Autodesk Inventor part; units mm, degrees
ref_plane "YZ Plane" through (0, 0, 0) normal (1, 0, 0) x (0, 1, 0)
ref_plane "XZ Plane" through (0, 0, 0) normal (0, 1, 0) x (-1, 0, 0)
ref_plane "XY Plane" through (0, 0, 0) normal (0, 0, 1) x (1, 0, 0)
sketch "スケッチ1" plane through (0, 0, 0) normal (0, 1, 0) x (-1, 0, 0)
  arc A0 (72.9254, -25.3463) -> (139.4294, -19.0858) centre (64.9013, 416.2515) ccw
  arc A1 (54.1052, -25.1311) -> (72.9254, -25.3463) centre (67.1484, 292.5868) ccw
  arc A2 (19.6951, -19.0145) -> (54.1052, -25.1311) centre (59.4352, 104.7024) ccw
  arc A3 (-0.0609, -9.311) -> (19.6951, -19.0145) centre (42.8692, 53.13) ccw
  arc A4 (-5.5029, -4.0266) -> (-0.0609, -9.311) centre (12.76, 9.3368) ccw
  arc A5 (-2.9938, 3.6874) -> (-5.5029, -4.0266) centre (-1.4678, -1.074) ccw
  arc A6 (5.1717, 4.7562) -> (-2.9938, 3.6874) centre (4.0256, -18.2153) ccw
  arc A7 (36.109, -0.9508) -> (5.1717, 4.7562) centre (-0.7578, -114.096) ccw
  arc A8 (36.109, -0.9508) -> (38.0145, -1.5673) centre (185.125, 456.3841) ccw
  arc A9 (38.0145, -1.5673) -> (139.3334, -17.8944) centre (142.307, 323.0926) ccw
  arc A10 (139.4294, -19.0858) -> (139.3334, -17.8944) centre (139.3282, -18.4944) ccw
  circle A11 centre (6.8478, -1.4519) radius 3
  circle A12 centre (92.934, -19.7045) radius 3
  point P0 (0, 0)
extrude "押し出し1" add sketch "スケッチ1" along normal mid plane 41.5
properties part number "uretan_s" material "ポリエチレン、高密度"
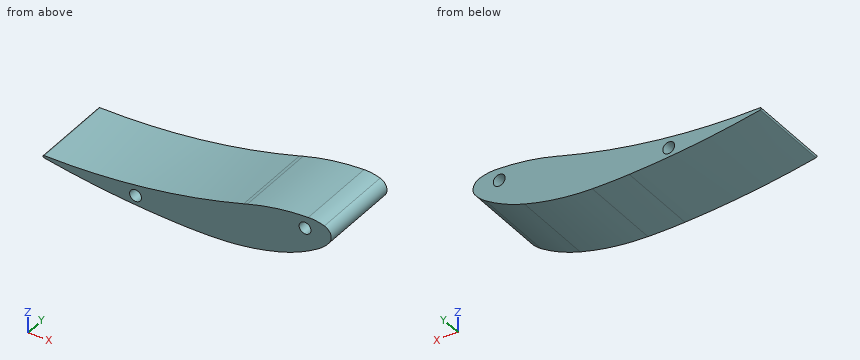
For this review, take the finished solid that the model builds, in its own axes (mm). Coordinates: 2 decimals unless noted, no trailing zeros. Order: outer loops, then holes, each group sorted by start corner. A loop starts at its lowest first (then second) coordinate and runs counter-clockwise, first axis right, second up. Notation, with made-up numbers: (63.5, 4) -> (111.5, 4) arc R14 cw to (111.5, 29) -> close; hole circle Ø11 at (66.25, 31). An arc over 180 degrees is marked (long way). Use CSV: the item, a comma, the result in double quotes. Start each with the question number.
Item 1: Wall thickness on probe 1 along Z at (x, y) = (-94, 10); probe 2 along Z at (x, y) = (-74, 1.5); probe 3 along Z at (x, y) = (-129, -18.5): over which ranges is each line inside the solid? List them lowest first.
Item 2: We need section C-C, the plane x = -125.5. Give the boundary of the cut face in (y, z).
Item 3: We need section A-A, the plane y = -4.5. Give the boundary of the cut face in (x, z), then the cut area to 3 significant figures.
Item 4: We need section B-B, the plane z = -21. Give the boundary of the cut face in (x, y), then the cut area to 3 significant figures.
Item 5: Insertion check: pin 1 (1 mm diameter, centred on x = -10, y = 5, fed in from -Z); pin 2 (12 mm diameter, centred on x = -72.5, y = -13.5, fed in from +Z). Each pin has a flat end and moves straight along its axis. Give the tip position at first contact, or say it passes through.
Item 6: We need section D-D, the plane z = -12. Give the boundary of the cut face in (x, y).
Derived:
1,probe 1,"z = -24.46 to -22.51, -16.9 to -14.47"
1,probe 2,"z = -25.33 to -11"
1,probe 3,"z = -20.74 to -17.65"
2,outline,"(-20.75, -21.24) -> (20.75, -21.24) -> (20.75, -17.49) -> (-20.75, -17.49) -> close"
3,outline,"(-139.43, -19.09) arc R441.67 ccw to (-72.93, -25.35) arc R318.06 ccw to (-54.11, -25.13) arc R129.94 ccw to (-19.7, -19.01) arc R75.77 ccw to (0.06, -9.31) arc R22.63 ccw to (5.5, -4.03) arc R5 ccw to (2.99, 3.69) arc R23 ccw to (-5.17, 4.76) arc R119 ccw to (-36.11, -0.95) arc R482.19 cw to (-38.01, -1.57) arc R341 cw to (-139.33, -17.89) arc R0.6 ccw to start; hole circle Ø6 at (-92.93, -19.7); hole circle Ø6 at (-6.85, -1.45)"
3,area,"1,940 mm^2"
4,outline,"(-127.22, -20.75) -> (-95.64, -20.75) -> (-95.64, 20.75) -> (-127.22, 20.75) -> close; (-90.23, -20.75) -> (-26.51, -20.75) -> (-26.51, 20.75) -> (-90.23, 20.75) -> close"
4,area,"3,960 mm^2"
5,pin 1,"stops at z = -15.38"
5,pin 2,"stops at z = -9.37"
6,outline,"(-79.11, -20.75) -> (-4.14, -20.75) -> (-4.14, 20.75) -> (-79.11, 20.75) -> close"
